from build123d import *

# Parameters (mm, degrees)
BOSS_EXTRUDE1_DEPTH  = 6.35
M5_CLEARANCE_HOLE1_D = 5.5
M4_CLEARANCE_HOLE1_D = 4.5
M5_CLEARANCE_HOLE2_D = 5.5


with BuildPart() as part:
    # Sketch1 → Boss-Extrude1 (new body)
    with BuildSketch(Plane.XY):
        with BuildLine():
            Line((0, 6.35), (101.6, 6.35))
            ThreePointArc((101.6, 6.35), (107.95, 0), (101.6, -6.35))
            Line((101.6, -6.35), (0, -6.35))
            ThreePointArc((0, -6.35), (-6.35, 0), (0, 6.35))
        make_face()
    extrude(amount=BOSS_EXTRUDE1_DEPTH)

    # M5 Clearance Hole1 (through all)
    with Locations(Plane(origin=(0, 0, 0), x_dir=(-1, 0, 0), z_dir=(0, 0, -1))):
        with Locations((-101.6, 0)):
            Hole(M5_CLEARANCE_HOLE1_D / 2)

    # M4 Clearance Hole1 (through all)
    with Locations(Plane(origin=(0, 0, 0), x_dir=(-1, 0, 0), z_dir=(0, 0, -1))):
        with Locations((-50.8, 0)):
            Hole(M4_CLEARANCE_HOLE1_D / 2)

    # M5 Clearance Hole2 (through all)
    with Locations(Plane.XY.offset(6.35)):
        with Locations((0, 0)):
            Hole(M5_CLEARANCE_HOLE2_D / 2)


solid = part.part
Can you work these out from the model? Positions are in its coordinate system, mm. Give positions to 0.01 mm unless a question says otherwise; leave off trailing zeros. Loops run counter-clockwise (first coordinate to the right, second up) from the corner with the lowest first, then second, coordinate; pieces in that order, holes last. Notation, with made-up numbers: (-18.75, 39) -> (40.25, 39) arc R7 ccw to (40.25, 49) -> close; hole circle Ø1 at (40, 31). An arc over 180 degrees is marked (long way). Return JSON: item names as keys, results as strings.
Q1. We'd pull the mould along Y, two halves only. Please class faces 1 (the face through (0.596, -2.685, 3.131)), 2 (the face through (104.22, 0.83, 3.22)), 3 (the face through (52, -6.35, 3)), 4 (the face through (50, 6.35, 3)): released by +Y, released by -Y, zero draft, split by the parting line, or undercut.
Checks:
{"face 1": "undercut", "face 2": "undercut", "face 3": "released by -Y", "face 4": "released by +Y"}
Q2. I want a section at A-A, the plane y = 0. List the corners of the cut face in (x, z) for me.
Checks:
{"outline": "(-6.35, 0) -> (-2.75, 0) -> (-2.75, 6.35) -> (-6.35, 6.35) -> close; (2.75, 0) -> (48.55, 0) -> (48.55, 6.35) -> (2.75, 6.35) -> close; (53.05, 0) -> (98.85, 0) -> (98.85, 6.35) -> (53.05, 6.35) -> close; (104.35, 0) -> (107.95, 0) -> (107.95, 6.35) -> (104.35, 6.35) -> close"}
Q3. I need wall thicknesses on probe 1 along Y at (x, z) = (101.6, 5.25); probe 2 along X at (y, z) = (1.5, 4). Which ranges of each line are inside material? Lowest first, please.
Checks:
{"probe 1": "y = -6.35 to -2.75, 2.75 to 6.35", "probe 2": "x = -6.17 to -2.3, 2.3 to 49.12, 52.48 to 99.3, 103.9 to 107.77"}
Q4. I want a section at C-C, the plane x = 50.8. List the corners of the cut face in (y, z) for me.
Checks:
{"outline": "(-6.35, 0) -> (-2.25, 0) -> (-2.25, 6.35) -> (-6.35, 6.35) -> close; (2.25, 0) -> (6.35, 0) -> (6.35, 6.35) -> (2.25, 6.35) -> close"}
Q5. I want a section at B-B, the plane z = 1.25. List the corners of the cut face in (x, y) for me.
Checks:
{"outline": "(0, -6.35) -> (101.6, -6.35) arc R6.35 ccw to (101.6, 6.35) -> (0, 6.35) arc R6.35 ccw to start; hole circle Ø5.5 at (0, 0); hole circle Ø4.5 at (50.8, 0); hole circle Ø5.5 at (101.6, 0)"}
